Here's how the part is built. I have some questions about the finished solid (model axes, mm). A direction names the side the tool comes from. Coordinates: 2 decimals unless noted, no trailing zeros. Loops run counter-clockwise (first coordinate to the right, second up) from the corner with the lowest first, then second, coordinate; pieces in that order, holes last. Notation, with made-up numbers: (58.5, -14) -> (103.5, -14) arc R8 ccw to (103.5, -5) -> close; hole circle Ø5 at (7, 7.25). An arc over 180 degrees is marked (long way). Answer as a JSON object with one key per item and string values. Group by question number.
1) I want a section at B-B (x = 0). Write out the boundary of the cut face in (y, z).
2) I want a section at C-C (x = -5). Write out the boundary of the cut face in (y, z).
3) I need wall thicknesses on probe 1 along X at (y, z) = (16.5, 0); probe 2 along Y at (x, z) = (3.75, -3). Which ranges of each line are inside material? Lowest first, please. Write a range as [from, to].
4) If we mould it in two halves opening along Z, with no side actions, what happens to faces 4 (the flat face through (0.19, 2.91, 5.62)), 5 (the cylindrical face through (-7.493, 18.675, 0.33)), 6 (the cylindrical face through (-0.46, 20.74, 3.52)), 7 (the flat face through (-5, 0, -3))? For each: +Z half, -Z half, draft (parallel to the pull), parting line (faces both ways), or undercut.
5) I want a section at A-A (y = 24). Write out the boundary of the cut face in (x, z), then the cut area to 3 significant figures.
6) I'm going to push flat-ended pins straight in: pin 1 (6 mm diameter, centred on y = 19, z = -3.5, fed in from -X); pin 2 (2 mm diameter, centred on y = 15, z = -4, fed in from -X); pin 3 (3.5 mm diameter, centred on x = 0.5, z = 1, fed in from -Y). Where does each tip first touch, or does it pass through?
7) Which directions (+Z, -Z, +X, -X, +Y, -Y) give clear straight access to the entire face, cutting with the end or side of a thin tool? Please do faces 1 (the flat face through (4.96, 2.91, 2.65)), 2 (the flat face through (0, 43.68, 0)), 3 (the cylindrical face through (0.518, 40.542, -3.946)).
Autodesk Fusion 360 part; units mm, degrees
sketch "Sketch1" plane through (0, 0, 0) normal (0, 1, 0) x (1, 0, 0)
  circle A0 centre (0, 0) radius 7.5
  line L0 (6.4897, 0.2677) -> (3.013, 5.7541)
  line L1 (3.013, 5.7541) -> (-3.4767, 5.4864)
  line L2 (-3.4767, 5.4864) -> (-6.4897, -0.2677)
  line L3 (-6.4897, -0.2677) -> (-3.013, -5.7541)
  line L4 (-3.013, -5.7541) -> (3.4767, -5.4864)
  line L5 (3.4767, -5.4864) -> (6.4897, 0.2677)
  circle A1 centre (0, 0) radius 3.55
  dimension "d1" = 15
  dimension "d2" = 5.625
  dimension "d7" = 7.1
extrude "Extrude1" add sketch "Sketch1" along normal blind 37.88 contours A0 | L0 L1 L2 L3 L4 L5 | A1
extrude "Extrude2" cut sketch "Sketch1" along normal blind 5.9 contours L0 L1 L2 L3 L4 L5 | A1
extrude "Extrude3" cut sketch "Sketch1" along normal blind 36 contours A1
sketch "Sketch2" plane through (0, 37.88, 0) normal (0, 1, 0) x (-1, 0, 0)
  circle A0 centre (0, 0) radius 7.5
  circle A1 centre (0, 0) radius 3.98
  dimension "d10" = 7.96
extrude "Extrude4" add sketch "Sketch2" along normal blind 5.8 contours A1
fillet "Fillet1" radius 0.4 1 edges at (3.7107, 43.68, -1.4392)
Determined:
{
 "1": {"outline": "(0, -7.5) -> (37.88, -7.5) -> (37.88, -3.98) -> (43.28, -3.98) arc R0.4 ccw to (43.68, -3.58) -> (43.68, 3.58) arc R0.4 ccw to (43.28, 3.98) -> (37.88, 3.98) -> (37.88, 7.5) -> (0, 7.5) -> (0, 5.63) -> (5.9, 5.63) -> (5.9, 3.55) -> (36, 3.55) -> (36, -3.55) -> (5.9, -3.55) -> (5.9, -5.63) -> (0, -5.63) -> close"},
 "2": {"outline": "(0, -5.59) -> (37.88, -5.59) -> (37.88, 5.59) -> (0, 5.59) -> (0, 2.62) -> (5.9, 2.62) -> (5.9, -2.58) -> (0, -2.58) -> close"},
 "3": {"probe 1": "[-7.5, -3.55], [3.55, 7.5]", "probe 2": "[5.9, 37.88]"},
 "4": {"face 4": "undercut", "face 5": "parting line", "face 6": "undercut", "face 7": "draft"},
 "5": {"outline": "circle Ø15 at (0, 0); hole circle Ø7.1 at (0, 0)", "area": "137 mm^2"},
 "6": {"pin 1": "x = -7.48", "pin 2": "x = -6.87", "pin 3": "y = 36"},
 "7": {"face 1": "-Y", "face 2": "+Z, -Z, +X, -X, +Y", "face 3": "+Y"}
}
